Build history of the part. All positions in model axes, mm. Round coordinates to 2 decimals unless told otherwise and drop trailing zeros. Write each loop counter-clockwise with the first axis right and the second up, starting at its lowest first coordinate (ties: lowest second). Pieces come first, ordered by that corner, then holes. Notation, with made-up numbers: (51.5, 0) -> (79.5, 0) arc R19 ccw to (79.5, 30) -> close; hole circle Ø1 at (19.5, 12.5). An arc over 180 degrees is marked (long way). One line per question, with ' | ' between items.
from build123d import *

# Parameters (mm, degrees)
SKETCH1_W           = 278
SKETCH1_H           = 100
BOSS_EXTRUDE1_DEPTH = 3
SKETCH2_W           = 40
SKETCH2_H           = 3
BOSS_EXTRUDE2_DEPTH = 3
SKETCH3_R           = 10.2
CUT_EXTRUDE1_DEPTH  = 3
SKETCH4_W           = 35
SKETCH4_H           = 3
SKETCH4_W_2         = 30
BOSS_EXTRUDE3_DEPTH = 3


with BuildPart() as part:
    # Sketch1 → Boss-Extrude1 (new body)
    with BuildSketch(Plane(origin=(0, 0, 0), x_dir=(1, 0, 0), z_dir=(0, 1, 0))):
        Rectangle(SKETCH1_W, SKETCH1_H)
    extrude(amount=BOSS_EXTRUDE1_DEPTH)

    # Sketch2 → Boss-Extrude2 (add)
    with BuildSketch(Plane(origin=(0, 0, -50), x_dir=(-1, 0, 0), z_dir=(0, 0, -1))):
        with Locations((-79, 1.5)):
            Rectangle(SKETCH2_W, SKETCH2_H)
        with Locations((-4, 1.5)):
            Rectangle(SKETCH2_W, SKETCH2_H)
        with Locations((79, 1.5)):
            Rectangle(SKETCH2_W, SKETCH2_H)
    extrude(amount=BOSS_EXTRUDE2_DEPTH)

    # Sketch3 → Cut-Extrude1 (cut)
    with BuildSketch(Plane(origin=(0, 3, 0), x_dir=(1, 0, 0), z_dir=(0, 1, 0))):
        with Locations(Location((72.4, 19.8, 0), (0, 0, 270))):
            Circle(SKETCH3_R)
        with Locations(Location((-78.8, -19.8, 0), (0, 0, 270))):
            Circle(SKETCH3_R)
        with Locations(Location((22, 19.8, 0), (0, 0, 270))):
            Circle(SKETCH3_R)
        with Locations(Location((-28.4, 19.8, 0), (0, 0, 270))):
            Circle(SKETCH3_R)
        with Locations(Location((-78.8, 19.8, 0), (0, 0, 270))):
            Circle(SKETCH3_R)
    extrude(amount=-CUT_EXTRUDE1_DEPTH, mode=Mode.SUBTRACT)

    # Sketch4 → Boss-Extrude3 (add)
    with BuildSketch(Plane.XY.offset(50)):
        with Locations((-87.5, 1.5)):
            Rectangle(SKETCH4_W, SKETCH4_H)
        with Locations((-20, 1.5)):
            Rectangle(SKETCH4_W_2, SKETCH4_H)
        with Locations((35, 1.5)):
            Rectangle(SKETCH4_W_2, SKETCH4_H)
        with Locations((90, 1.5)):
            Rectangle(SKETCH4_W_2, SKETCH4_H)
    extrude(amount=BOSS_EXTRUDE3_DEPTH)


solid = part.part
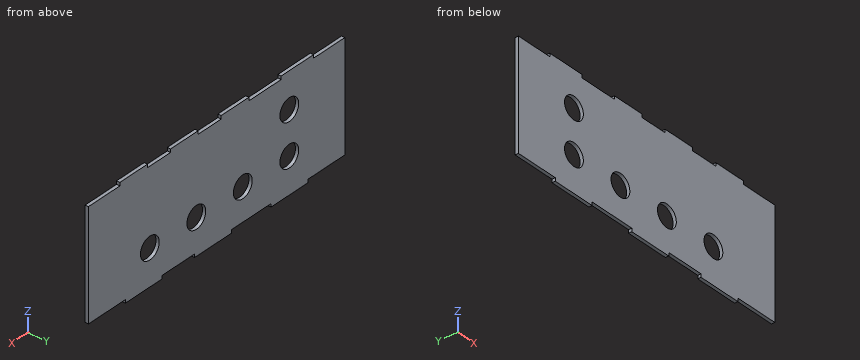
(1) Slice it at C-C (z = -19.8). Write the cut outline in (x, y).
Calculated:
outline: (-139, 0) -> (-89, 0) -> (-89, 3) -> (-139, 3) -> close; (-68.6, 0) -> (-38.6, 0) -> (-38.6, 3) -> (-68.6, 3) -> close; (-18.2, 0) -> (11.8, 0) -> (11.8, 3) -> (-18.2, 3) -> close; (32.2, 0) -> (62.2, 0) -> (62.2, 3) -> (32.2, 3) -> close; (82.6, 0) -> (139, 0) -> (139, 3) -> (82.6, 3) -> close
(2) Wall check: line 1 (X direction, y = 1.85, z = -19.8); line 2 (X direction, y = 1.85, z = 19.8); line 3 (X direction, y = 2.1, z = -21.5). Give the ranges that are in metal, low to high. Write a range as from..to.
Calculated:
line 1: -139..-89, -68.6..-38.6, -18.2..11.8, 32.2..62.2, 82.6..139 | line 2: -139..-89, -68.6..139 | line 3: -139..-88.86, -68.74..-38.46, -18.34..11.94, 32.06..62.34, 82.46..139
(3) Slice it at D-D (y = 0.95). State how many separate pieces and enclosed holes the cut face has, then the cut area to 3 significant figures.
Calculated:
separate pieces: 1 | enclosed holes: 5 | area: 26,900 mm2
(4) Slice it at B-B (x = -28.4). Write the cut outline in (y, z).
Calculated:
outline: (0, -50) -> (3, -50) -> (3, -30) -> (0, -30) -> close; (0, -9.6) -> (3, -9.6) -> (3, 53) -> (0, 53) -> close
(5) Slice it at A-A (z = 19.8). Write the cut outline in (x, y), then the cut area to 3 significant figures.
Calculated:
outline: (-139, 0) -> (-89, 0) -> (-89, 3) -> (-139, 3) -> close; (-68.6, 0) -> (139, 0) -> (139, 3) -> (-68.6, 3) -> close | area: 773 mm2
(6) Drop flat-ended pins along their axis: pin 1 (0.9 mm diameter, centred on y = 2, z = 52, fed in from -X); pin 2 (1.5 mm diameter, centred on y = 2, z = 51, fed in from +X); pin 3 (0.9 mm diameter, centred on x = 117, y = 1.5, fed in from -Z). Give the stop position or say it passes through.
Calculated:
pin 1: x = -105 | pin 2: x = 105 | pin 3: z = -50
